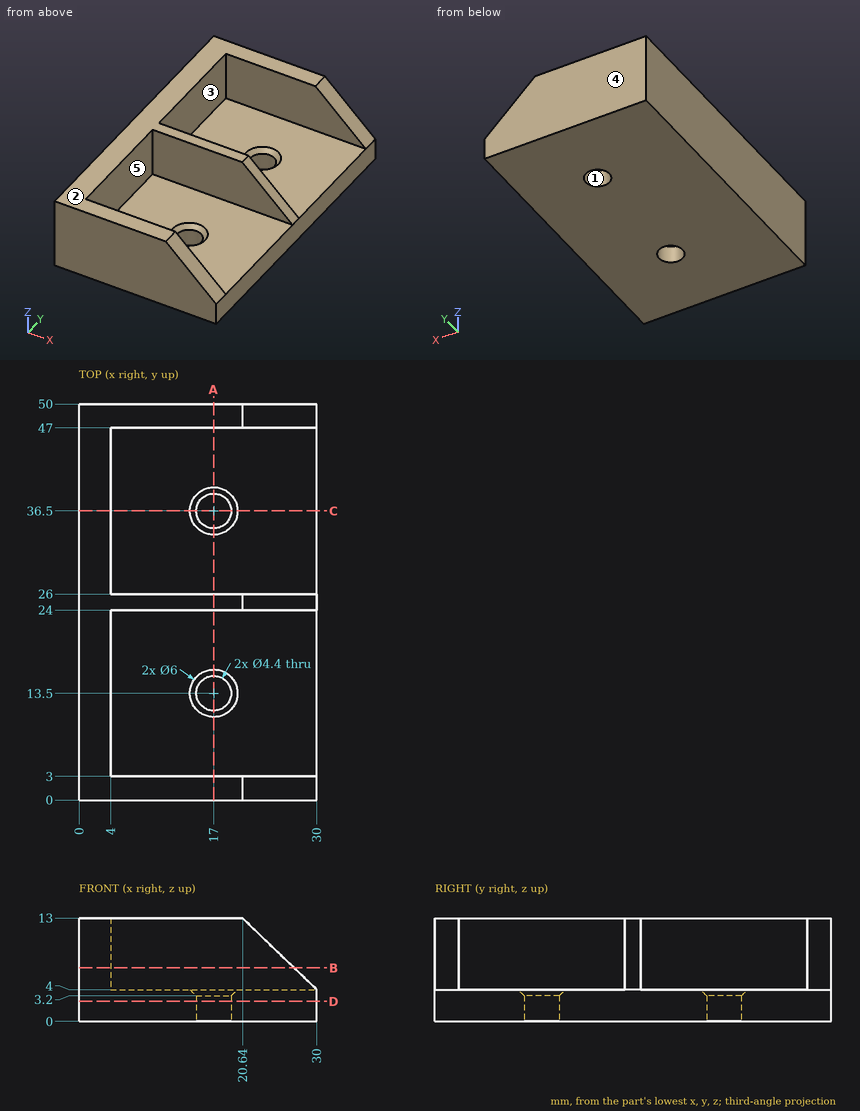
For this review, use the dimensioned drawing (mm, ordinates from the lowest corner) and the shaded views. A direction names the side the tool comes from. Coordinates: 2 decimals unless noted, no trailing zeros. Loops run counter-clockwise (first coordinate to the right, second up) from the corner with the lowest first, then second, coordinate; pieces in that order, holes last. Notation, with made-up numbers: (8.25, 46.5) - (41.25, 46.5) arc R17 cw to (41.25, 61.5) - close; hole circle Ø5 at (-22.75, 87.25). An arc over 180 degrees is marked (long way). Use CSV: the item, a comma, the result in double quotes. Start each with the question number.
1) Tool access review of the marked faces 4 and 5: name each direction out of +Z, -Z, +X, -X, +Y, -Y from which nothing blocks a thin tool from reaching the whole face with its end or side.
2) Consider section A-A on x = 17. Write out the cut boundary in (y, z).
3) The part is to be moulded in two halves that separate along X. For the marked faces 1, 2 and 3, say which applies: +X half, -X half, draft (parallel to the pull), parting line (faces both ways), or undercut.
4) Wall thickness on L1, parallel to Y at x = 17, z = 0.7; L2, parallel to Y at x = 13, z = 8.25; L3, parallel to X at y = 36.5, z = 1.95: over which ranges is each line inside the solid? List them lowest first. Write a range as from..to.
5) Consider section B-B on z = 6.75. Write out the cut boundary in (x, y), then the cut area to 3 significant figures.
6) Consider section D-D on z = 2.5. Write out the cut boundary in (x, y).
7) Consider section C-C on y = 36.5. Write out the cut boundary in (x, z).
8) For pin 1 Ø3 at (x, y) = (7.5, 8.5) entering from +Z; pin 2 Ø4.5 at (y, z) = (31.5, 8) entering from +X; pin 3 Ø2.5 at (x, y) = (17, 36.5) entering from -Z; pin 4 Ø5.5 at (x, y) = (17, 13.5) entering from +Z, all flat-tipped, find the tip position at first contact; note any pin that passes through.
Geometry says:
1,face 4,"+Z, -Z, +X, -X, +Y"
1,face 5,"+Z, +X"
2,outline,"(0, 0) - (11.3, 0) - (11.3, 3.2) - (10.5, 4) - (3, 4) - (3, 13) - (0, 13) - close; (15.7, 0) - (34.3, 0) - (34.3, 3.2) - (33.5, 4) - (26, 4) - (26, 13) - (24, 13) - (24, 4) - (16.5, 4) - (15.7, 3.2) - close; (38.7, 0) - (50, 0) - (50, 13) - (47, 13) - (47, 4) - (39.5, 4) - (38.7, 3.2) - close"
3,face 1,"undercut"
3,face 2,"draft"
3,face 3,"+X half"
4,L1,"0..11.3, 15.7..34.3, 38.7..50"
4,L2,"0..3, 24..26, 47..50"
4,L3,"0..14.8, 19.2..30"
5,outline,"(0, 0) - (27.14, 0) - (27.14, 3) - (4, 3) - (4, 24) - (27.14, 24) - (27.14, 26) - (4, 26) - (4, 47) - (27.14, 47) - (27.14, 50) - (0, 50) - close"
5,area,"385 mm^2"
6,outline,"(0, 0) - (30, 0) - (30, 50) - (0, 50) - close; hole circle Ø4.4 at (17, 13.5); hole circle Ø4.4 at (17, 36.5)"
7,outline,"(0, 0) - (14.8, 0) - (14.8, 3.2) - (14, 4) - (4, 4) - (4, 13) - (0, 13) - close; (19.2, 0) - (30, 0) - (30, 4) - (20, 4) - (19.2, 3.2) - close"
8,pin 1,"z = 4"
8,pin 2,"x = 4"
8,pin 3,"through"
8,pin 4,"z = 3.75"
